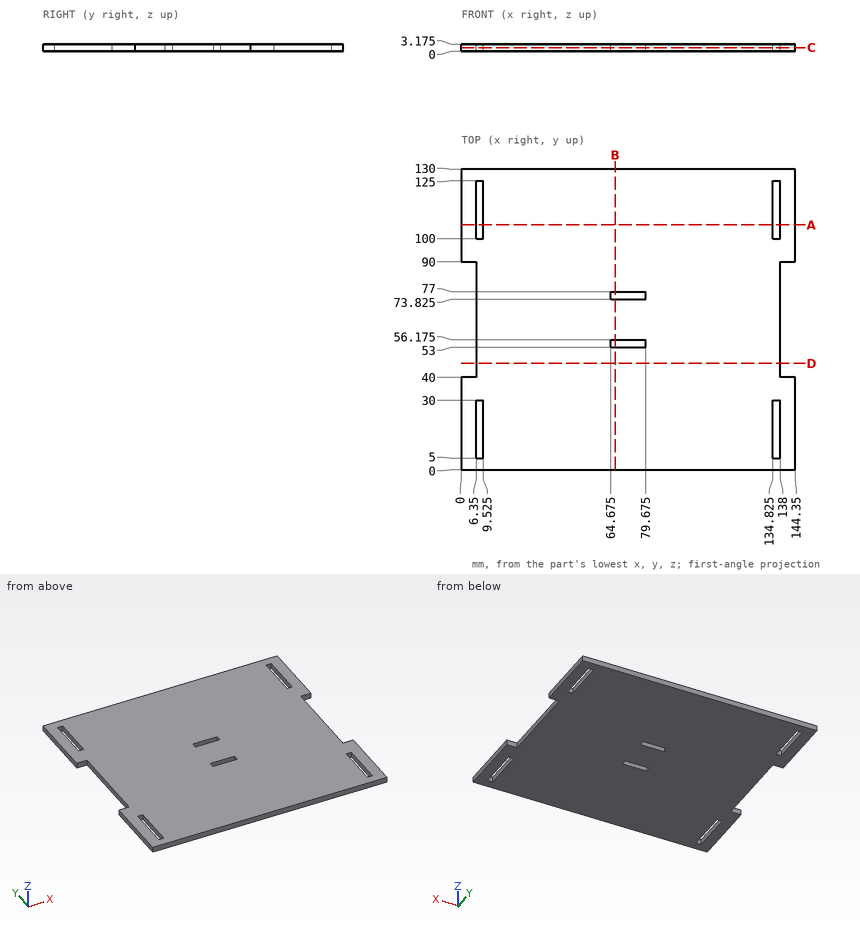
Here's the drawing with two shaded views (mm, measured from the low corner). I have some questions. Coordinates: 2 decimals unless noted, no trailing zeros. Order: outer loops, then holes, each group sorted by start corner. A loop starts at its lowest first (then second) coordinate and runs counter-clockwise, first axis right, second up. Notation, with made-up numbers: (72, 86) -> (93, 86) arc R28 ccw to (93, 123) -> close; hole circle Ø3 at (1, 62.5). An arc over 180 degrees is marked (long way). Write each question's results on one line, items separated by ' | '.
Item 1: I want a section at A-A, the plane y = 106. Write out the boundary of the cut face in (x, z) (3 decimals).
Results are:
outline: (0, 0) -> (6.35, 0) -> (6.35, 3.175) -> (0, 3.175) -> close; (9.525, 0) -> (134.825, 0) -> (134.825, 3.175) -> (9.525, 3.175) -> close; (138, 0) -> (144.35, 0) -> (144.35, 3.175) -> (138, 3.175) -> close
Item 2: I'm going to push flat-ended pins straight in: pin 1 Ø1.6 at (x, z) = (8.5, 2) entering from -Y; pin 2 Ø1 at (y, z) = (74.5, 2.5) entering from -X. Where does each tip first touch, or does it pass through?
Results are:
pin 1: y = 0 | pin 2: x = 6.35
Item 3: I want a section at D-D, the plane y = 46. Write out the boundary of the cut face in (x, z) (3 decimals).
Results are:
outline: (6.35, 0) -> (138, 0) -> (138, 3.175) -> (6.35, 3.175) -> close
Item 4: If I drill on line 1 along Y through (x, z) = (78, 1.5) (3 decimals); line 2 along X through (y, z) = (122, 2.4) (3 decimals); line 3 along X through (y, z) = (73.5, 1.8), over which ranges is the centre line in solid material (lowest first)?
Results are:
line 1: 0 to 53, 56.175 to 73.825, 77 to 130 | line 2: 0 to 6.35, 9.525 to 134.825, 138 to 144.35 | line 3: 6.35 to 138
Item 5: I want a section at C-C, the plane z = 1.6. Count the separate pieces of the cut face and the enclosed holes in it, then the cut area to 3 significant figures.
Results are:
separate pieces: 1 | enclosed holes: 6 | area: 17,700 mm²
Item 6: I want a section at B-B, the plane x = 66.5. Write out the boundary of the cut face in (y, z) (3 decimals).
Results are:
outline: (0, 0) -> (53, 0) -> (53, 3.175) -> (0, 3.175) -> close; (56.175, 0) -> (73.825, 0) -> (73.825, 3.175) -> (56.175, 3.175) -> close; (77, 0) -> (130, 0) -> (130, 3.175) -> (77, 3.175) -> close
